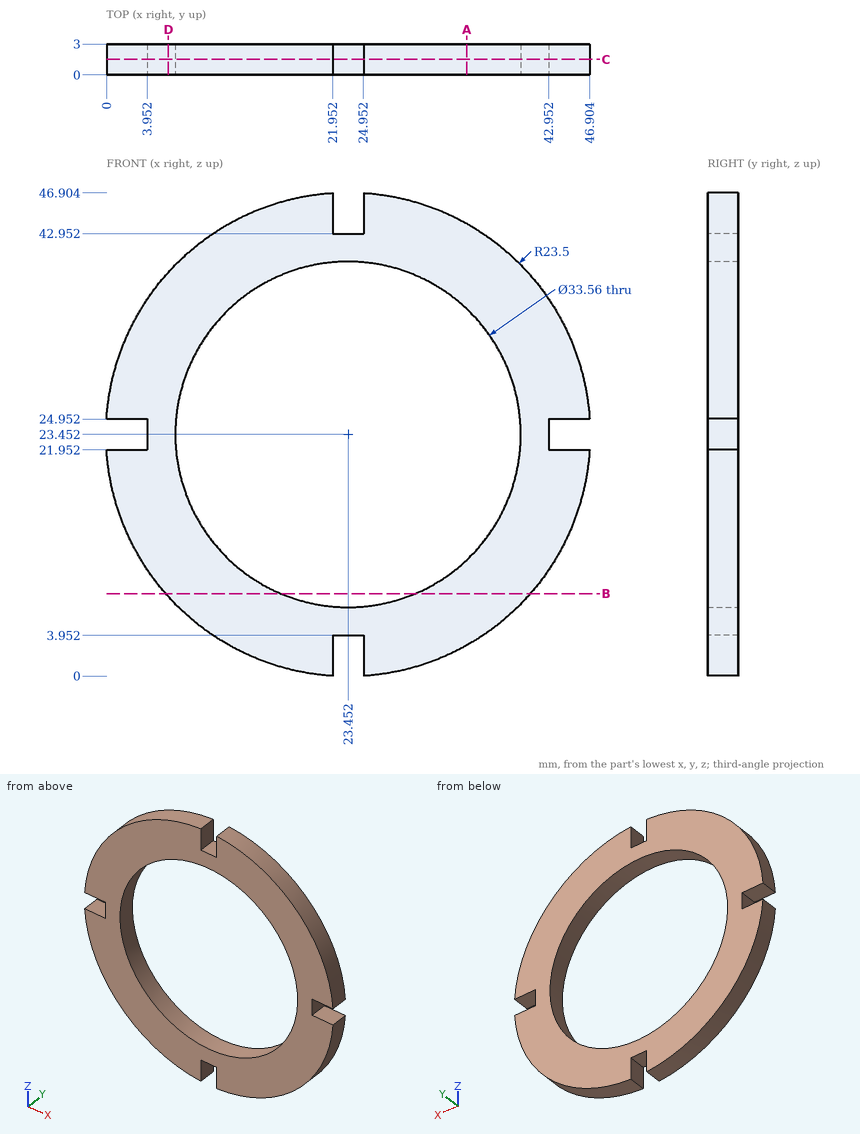
Could you check a few things on this drawing? It's one solid part, dimensions in mm from its lowest x, y, z. Coordinates: 2 decimals unless noted, no trailing zeros. Order: outer loops, then holes, each group sorted by start corner. A loop starts at its lowest first (then second) coordinate and runs counter-clockwise, first axis right, second up. Notation, with made-up numbers: (76, 12.5) - (109, 12.5) arc R19 cw to (109, 17.5) - close; hole circle Ø8 at (77, 14). An arc over 180 degrees is marked (long way). Answer as a JSON object with one key per item and string values. Group by question number.
Q1. Imagine slicing it at C-C (y = 1.5). Please give me the cut outline in (x, z).
Q2. Imagine slicing it at A-A (x = 35). Please give me the cut outline in (y, z) (1 decimal).
Q3. Will these pins go through, and if not, where does the flat tip stop? P1, Ø0.9, axis at y = 1, z = 2, coming from the +X side (1 decimal); P2, Ø1.5, axis at y = 1.5, z = 1.5, coming from the -X side; P3, Ø1.5, axis at y = 1, z = 44, coming from the +X side.
Q4. Imagine slicing it at D-D (x = 6). Please give me the cut outline in (y, z).
Q5. Imagine slicing it at B-B (z = 8). Please give me the cut outline in (x, y).
Q6. I need wall thicknesses on line 1 (Z direction, x = 11.5, y = 2.35) (1 decimal); line 2 (Z direction, x = 15.5, y = 0.6); line 3 (X direction, y = 0.2, z = 26.5). Which ranges of each line are inside material? Lowest first, please. Write a range as from..to.
Determined:
{
 "1": {"outline": "(0, 21.95) arc R23.5 ccw to (21.95, 0) - (21.95, 3.95) - (24.95, 3.95) - (24.95, 0) arc R23.5 ccw to (46.9, 21.95) - (42.95, 21.95) - (42.95, 24.95) - (46.9, 24.95) arc R23.5 ccw to (24.95, 46.9) - (24.95, 42.95) - (21.95, 42.95) - (21.95, 46.9) arc R23.5 ccw to (0, 24.95) - (3.95, 24.95) - (3.95, 21.95) - close; hole circle Ø33.56 at (23.45, 23.45)"},
 "2": {"outline": "(0, 3) - (3, 3) - (3, 11.3) - (0, 11.3) - close; (0, 35.6) - (3, 35.6) - (3, 43.9) - (0, 43.9) - close"},
 "3": {"P1": "stops at x = 34", "P2": "stops at x = 13.32", "P3": "stops at x = 36.11"},
 "4": {"outline": "(0, 7.71) - (3, 7.71) - (3, 39.19) - (0, 39.19) - close"},
 "5": {"outline": "(5.75, 0) - (16.91, 0) - (16.91, 3) - (5.75, 3) - close; (29.99, 0) - (41.16, 0) - (41.16, 3) - (29.99, 3) - close"},
 "6": {"line 1": "z = 3.2..11.7, 35.2..43.7", "line 2": "z = 1.34..8.68, 38.23..45.57", "line 3": "x = 0.15..6.95, 39.95..46.75"}
}
